Autodesk Inventor part; units mm, degrees
ref_plane "YZ Plane" through (0, 0, 0) normal (1, 0, 0) x (0, 1, 0)
ref_plane "XZ Plane" through (0, 0, 0) normal (0, 1, 0) x (-1, 0, 0)
ref_plane "XY Plane" through (0, 0, 0) normal (0, 0, 1) x (1, 0, 0)
sketch "Sketch1" plane through (0, 0, 0) normal (0, 1, 0) x (-1, 0, 0)
  circle A0 centre (0, 0) radius 1.5
  line L0 (-0.7211, -2.912) -> (-2.8825, -0.8315)
  line L1 (-2.8825, -0.8315) -> (-2.1614, 2.0805)
  line L2 (-2.1614, 2.0805) -> (0.7211, 2.912)
  line L3 (0.7211, 2.912) -> (2.8825, 0.8315)
  line L4 (2.8825, 0.8315) -> (2.1614, -2.0805)
  line L5 (2.1614, -2.0805) -> (-0.7211, -2.912)
  dimension "d0" = 3
  dimension "d1" = 6
extrude "Extrusion1" add sketch "Sketch1" along normal blind 60
thread "Thread1"
thread "Thread2"
properties part number "Spacer60"
Could you check a few things on this model? Use its own coordinates, in mm. Round coordinates to 2 decimals unless told otherwise and drop trailing zeros. Order: outer loops, then holes, each group sorted by start corner. A loop starts at its lowest first (then second) coordinate and runs counter-clockwise, first axis right, second up.
(1) Please list where these lines run through material, in increasing order: line 1 along Z through (x, y) = (-0.5, 14.5); line 2 along X through (y, z) = (35, -0.2); line 3 along Z through (x, y) = (0, 22).
Response values:
line 1: z = -2.56 to -1.41, 1.41 to 2.85
line 2: x = -2.63 to -1.49, 1.49 to 2.73
line 3: z = -2.7 to -1.5, 1.5 to 2.7
(2) If we mould it in two halves opening along Z, with no side actions, what happens to faces 1 (the flat face through (2.53, 29.58, 0.6)), 2 (the cylindrical face through (1.5, 29.58, -0.07)), 3 (the flat face through (-1.2, 0, -1.3))? For each: released by +Z, released by -Z, zero draft, split by the parting line, or undercut.
Response values:
face 1: released by +Z
face 2: undercut
face 3: zero draft
(3) Imagine slicing it at A-A (y = 39.5). Write out the boundary of the cut face in (x, z).
Response values:
outline: (-2.88, 0.83) - (-2.16, -2.08) - (0.72, -2.91) - (2.88, -0.83) - (2.16, 2.08) - (-0.72, 2.91) - close; hole circle Ø3 at (0, 0)
(4) I'm going to push flat-ended pins straight in: pin 1 (2 mm diameter, centred on y = 39.5, z = -1, fed in from -X); pin 2 (2 mm diameter, centred on x = -1.5, y = 34, fed in from -Z). Where does each tip first touch, or does it pass through?
Response values:
pin 1: stops at x = -2.68
pin 2: stops at z = -2.56
(5) Imagine slicing it at B-B (x = 0.15). Write out the boundary of the cut face in (y, z), plus the area to 3 significant figures.
Response values:
outline: (0, -2.75) - (60, -2.75) - (60, -1.49) - (0, -1.49) - close; (0, 1.49) - (60, 1.49) - (60, 2.66) - (0, 2.66) - close
area: 145 mm2
(6) Imagine slicing it at C-C (z = 0). Write out the boundary of the cut face in (x, y), plus the area to 3 significant figures.
Response values:
outline: (-2.68, 0) - (-1.5, 0) - (-1.5, 60) - (-2.68, 60) - close; (1.5, 0) - (2.68, 0) - (2.68, 60) - (1.5, 60) - close
area: 141 mm2
